The model under review builds one solid part; all positions refer to its coordinate system, in mm. A direction names the side the tool comes from. Give positions to 0.01 mm unless a question says otherwise; leave off trailing zeros. Loops run counter-clockwise (first coordinate to the right, second up) from the corner with the lowest first, then second, coordinate; pieces in that order, holes last. Notation, with made-up numbers: (-30, 69) - (8, 69) arc R21 ccw to (8, 91) - close; hole circle Ø11 at (70, -29.75). An arc over 180 degrees is marked (long way). Return JSON: item names as keys, results as strings. Group by question number.
```python
from build123d import *

# Parameters (mm, degrees)
BOX_W        = 10
BOX_H        = 10
BOX_DEPTH    = 10
BOX001_W     = 10
BOX001_H     = 10
BOX001_DEPTH = 3


with BuildPart() as cube:
    # Box → Box (new body)
    with BuildSketch(Plane.XY):
        with Locations((5, 5)):
            Rectangle(BOX_W, BOX_H)
    extrude(amount=BOX_DEPTH)


with BuildPart() as fusion:
    # Box001 → Box001 (new body)
    with BuildSketch(Plane(origin=(10, 0, 0), x_dir=(1, 0, 0), z_dir=(0, 0, 1))):
        with Locations((5, 5)):
            Rectangle(BOX001_W, BOX001_H)
    extrude(amount=BOX001_DEPTH)

    # Fusion: union Cube
    add(cube.part)


solid = fusion.part
```
1) For pin 1 Ø1 at (x, y) = (7.5, 2) entering from -Z; pin 2 Ø3 at (y, z) = (3, 5.5) entering from +X; pin 3 Ø6 at (x, y) = (13.5, 7.5) entering from +Z, all flat-tipped, find the tip position at first contact; note any pin that passes through.
2) We need section B-B, the plane z = 5. Write out the cut boundary in (x, y), plus the area to 3 significant figures.
3) To check wall thickness, follow line 1 (X direction, y = 6.25, z = 6); line 2 (Z direction, x = 11.75, y = 9.75). State the ranges of each line that lie inside material, in increasing order.
4) Tool access review of faces 1 (the face through (5, 5, 10)), 2 (the face through (10, 5, 6)): name each direction out of +Z, -Z, +X, -X, +Y, -Y from which nothing blocks a thin tool from reaching the whole face with its end or side.
5) We need section C-C, the plane x = 16.5. Write out the cut boundary in (y, z), plus the area to 3 significant figures.
6) We need section A-A, the plane y = 1.75. Write out the cut boundary in (x, z), plus the area to 3 significant figures.
Findings:
{
 "1": {"pin 1": "stops at z = 0", "pin 2": "stops at x = 10", "pin 3": "stops at z = 3"},
 "2": {"outline": "(0, 0) - (10, 0) - (10, 10) - (0, 10) - close", "area": "100 mm^2"},
 "3": {"line 1": "x = 0 to 10", "line 2": "z = 0 to 3"},
 "4": {"face 1": "+Z, +X, -X, +Y, -Y", "face 2": "+Z, +X, +Y, -Y"},
 "5": {"outline": "(0, 0) - (10, 0) - (10, 3) - (0, 3) - close", "area": "30.0 mm^2"},
 "6": {"outline": "(0, 0) - (20, 0) - (20, 3) - (10, 3) - (10, 10) - (0, 10) - close", "area": "130 mm^2"}
}
